from build123d import *

# Parameters (mm, degrees)
CROQUIS1_R              = 12.5
SALIENTE_EXTRUIR1_DEPTH = 2
REDONDEO2_R             = 1
CROQUIS2_R              = 5
SALIENTE_EXTRUIR2_DEPTH = 33.41
CROQUIS3_R              = 1.5
CORTAR_EXTRUIR1_DEPTH   = 23.41
CORTAR_EXTRUIR2_START   = -10
CORTAR_EXTRUIR2_DEPTH   = 10
CORTAR_EXTRUIR7_START   = -33.41
CROQUIS9_R              = 5
CROQUIS9_R_2            = 4.7
CORTAR_EXTRUIR7_DEPTH   = 33.41


with BuildPart() as part:
    # Croquis1 → Saliente-Extruir1 (new body)
    with BuildSketch(Plane.XY):
        Circle(CROQUIS1_R)
    extrude(amount=SALIENTE_EXTRUIR1_DEPTH)

    # Redondeo2
    redondeo2_edges = [part.edges().sort_by_distance(p)[0] for p in [
        (-12.5, 0, 2),
    ]]
    fillet(redondeo2_edges, radius=REDONDEO2_R)

    # Croquis2 → Saliente-Extruir2 (add)
    with BuildSketch(Plane(origin=(0, 0, 0), x_dir=(-1, 0, 0), z_dir=(0, 0, -1))):
        Circle(CROQUIS2_R)
    extrude(amount=SALIENTE_EXTRUIR2_DEPTH)

    # Croquis3 → Cortar-Extruir1 (cut)
    with BuildSketch(Plane(origin=(0, 0, 0), x_dir=(-1, 0, 0), z_dir=(0, 0, -1))):
        with Locations((0, 8.62)):
            Circle(CROQUIS3_R)
        with Locations((-8.62, 0)):
            Circle(CROQUIS3_R)
        with Locations((8.7, 0)):
            Circle(CROQUIS3_R)
        with Locations((0, -8.62)):
            Circle(CROQUIS3_R)
    extrude(amount=-CORTAR_EXTRUIR1_DEPTH, mode=Mode.SUBTRACT)

    # Croquis4 → Cortar-Extruir2 (cut)
    with BuildSketch(Plane(origin=(0, 0, -33.41), x_dir=(-1, 0, 0), z_dir=(0, 0, -1)).offset(CORTAR_EXTRUIR2_START)):
        with BuildLine():
            Line((-1, 4.898979486), (-1, 1.732050808))
            ThreePointArc((-1, 1.732050808), (-1.547786782, -1.266631784), (1.5, -1.322875656))
            Line((1.5, -1.322875656), (1.5, 1.322875656))
            ThreePointArc((1.5, 1.322875656), (1.266631784, 1.547786782), (1, 1.732050808))
            Line((1, 1.732050808), (1, 4.898979486))
            ThreePointArc((1, 4.898979486), (0, 5), (-1, 4.898979486))
        make_face()
    extrude(amount=CORTAR_EXTRUIR2_DEPTH, mode=Mode.SUBTRACT)

    # Croquis9 → Cortar-Extruir7 (cut)
    with BuildSketch(Plane(origin=(0, 0, -33.41), x_dir=(-1, 0, 0), z_dir=(0, 0, -1)).offset(CORTAR_EXTRUIR7_START)):
        Circle(CROQUIS9_R)
        with Locations(Location((0, 0, 0), (0, 0, 77.715506144))):
            Circle(CROQUIS9_R_2, mode=Mode.SUBTRACT)
    extrude(amount=CORTAR_EXTRUIR7_DEPTH, mode=Mode.SUBTRACT)


solid = part.part
For this review, take the finished solid that the model builds, in its own axes (mm). A direction names the side the tool comes from. Coordinates: 2 decimals unless noted, no trailing zeros. Loops run counter-clockwise (first coordinate to the right, second up) from the corner with the lowest first, then second, coordinate; pieces in that order, holes last. Notation, with made-up numbers: (49.25, 46) - (53.25, 46) arc R26 cw to (53.25, 79) - close; hole circle Ø4 at (6, 55). An arc over 180 degrees is marked (long way). Return JSON: item names as keys, results as strings.
Item 1: Take a section at B-B (z = -15). Give the boundary of the cut face in (x, y), then the cut area to 3 significant figures.
Determined:
{"outline": "circle Ø9.4 at (0, 0)", "area": "69.4 mm2"}
Item 2: Take a section at A-A (x = 0). Give the boundary of the cut face in (y, z).
Determined:
{"outline": "(-12.5, 0) - (-10.12, 0) - (-10.12, 2) - (-11.5, 2) arc R1 ccw to (-12.5, 1) - close; (-7.12, 0) - (-4.7, 0) - (-4.7, -33.41) - (-2, -33.41) - (-2, -23.41) - (4.7, -23.41) - (4.7, 0) - (7.12, 0) - (7.12, 2) - (-7.12, 2) - close; (10.12, 0) - (12.5, 0) - (12.5, 1) arc R1 ccw to (11.5, 2) - (10.12, 2) - close"}
Item 3: Insertion check: pin 1 (2 mm diameter, centred on y = -0.5, z = -26.5, fed in from +X); pin 2 (1 mm diameter, centred on x = 0, y = 1.5, fed in from -Z); pin 3 (3 mm diameter, centred on y = 3.5, z = -30, fed in from +X); pin 4 (2.5 mm diameter, centred on x = 0, y = -8.62, fed in from -Z). Each pin has a flat end and moves straight along its axis. Give the tip position at first contact, or say it passes through.
Determined:
{"pin 1": "stops at x = 4.7", "pin 2": "stops at z = -23.41", "pin 3": "stops at x = 4.25", "pin 4": "passes through"}
Item 4: For faces 1 (the flat face through (1, 3, -28)), 2 (the cylindrical face through (1.6, -1.2, -28.3)), 3 (the cylindrical face through (11.923, 3.755, 0.493)), list the 3-axis set-ups (+Z, -Z, +X, -X, +Y, -Y) from which the entire face can be reached by the end or side of a thin tool; tool diameter is ignored.
Determined:
{"face 1": "-Z, +Y", "face 2": "-Z", "face 3": "+Z, -Z"}
Item 5: Mouldability with a two-part tool opening along Y and no side actions: class faces 4 (the flat face through (0, 1, -23.41)), 5 (the cylindrical face through (-2.001, -4.253, -16.471)), 6 (the flat face through (-1, -2, -33.41)) as pulls with the +Y half, pulls with the -Y half, needs draft (parallel to the pull), parting line crosses it, or undercut.
Determined:
{"face 4": "undercut", "face 5": "parting line crosses it", "face 6": "needs draft"}
Item 6: For line 1 (Y direction, x = 0, z = 1.1); line 2 (Z direction, x = -4.5, y = 3); line 3 (X direction, y = -1.75, z = -23.5), list the stretches that pass through material, from the lowest coordinate up.
Determined:
{"line 1": "y = -12.49 to -10.12, -7.12 to 7.12, 10.12 to 12.49", "line 2": "z = 0 to 2", "line 3": "x = -4.36 to -0.97, 0.97 to 4.36"}
